Design review of the part shown in the three views and the two pictorial views. Dimensions are in mm from the part's minimum x, y and z. Round coordinates to 2 decimals unless told otherwise and drop trailing zeros. Loops run counter-clockwise (first coordinate to the right, second up) from the corner with the lowest first, then second, coordinate; pieces in that order, holes last. Notation, with made-up numbers: (71, 2.5) -> (121, 2.5) arc R23 cw to (121, 40.5) -> close; hole circle Ø5 at (19.25, -18.5). An arc over 180 degrees is marked (long way). Use a Markdown table: item, result. Add a question column.
1) Insertion check: pin 1 (1.5 mm diameter, centred on x = 125.5, y = 15, fed in from -Z). The pin has a flat end and moves straight along its axis. Give the tip position at first contact, or say it passes through.
2) Wall thickness on probe 1 along Y at (x, z) = (198.5, 0.5); probe 2 along X at (y, z) = (30, 2.25); probe 3 along X at (y, z) = (14, 4.2): over which ranges is each line inside the solid? List them lowest first.
3) Consider section C-C on x = 185. Give the boundary of the cut face in (y, z), plus the area to 3 significant figures.
4) Consider section B-B on y = 14. Give the boundary of the cut face in (x, z), plus the area to 3 significant figures.
5) Consider section A-A on z = 1.4. Give the boundary of the cut face in (x, y).
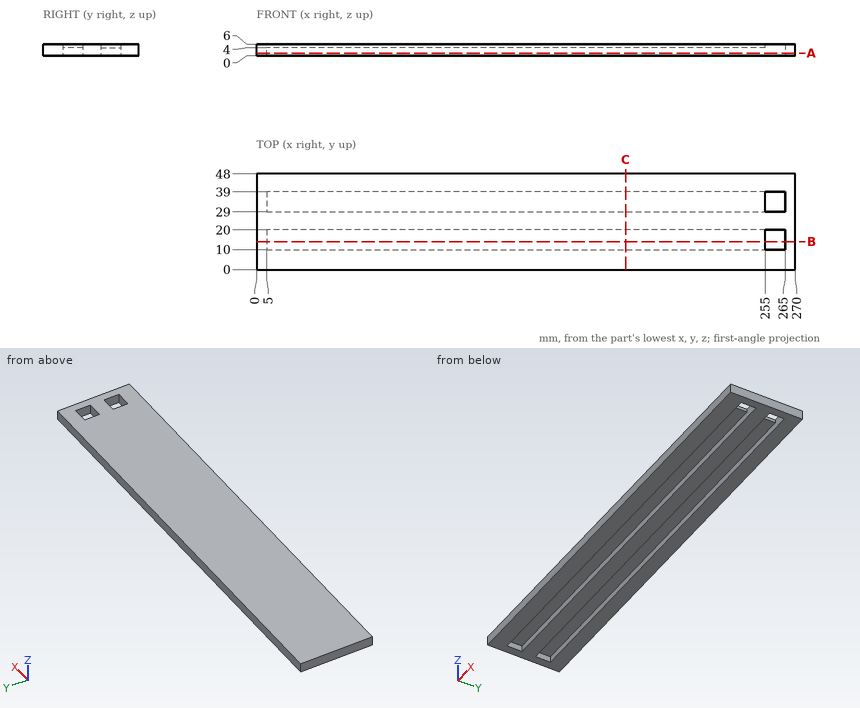
Result set:
| question | item | result |
|---|---|---|
| 1 | pin 1 | z = 4 |
| 2 | probe 1 | 0 to 10, 20 to 29, 39 to 48 |
| 2 | probe 2 | 0 to 5, 265 to 270 |
| 2 | probe 3 | 0 to 255, 265 to 270 |
| 3 | outline | (0, 0) -> (10, 0) -> (10, 4) -> (20, 4) -> (20, 0) -> (29, 0) -> (29, 4) -> (39, 4) -> (39, 0) -> (48, 0) -> (48, 6) -> (0, 6) -> close |
| 3 | area | 208 mm2 |
| 4 | outline | (0, 0) -> (5, 0) -> (5, 4) -> (255, 4) -> (255, 6) -> (0, 6) -> close; (265, 0) -> (270, 0) -> (270, 6) -> (265, 6) -> close |
| 4 | area | 560 mm2 |
| 5 | outline | (0, 0) -> (270, 0) -> (270, 48) -> (0, 48) -> close; hole (5, 10) -> (265, 10) -> (265, 20) -> (5, 20) -> close; hole (5, 29) -> (265, 29) -> (265, 39) -> (5, 39) -> close |
